Build history of the part. All positions in model axes, mm. A direction names the side the tool comes from. Give positions to 0.01 mm unless a question says otherwise; leave off trailing zeros. Loops run counter-clockwise (first coordinate to the right, second up) from the corner with the lowest first, then second, coordinate; pieces in that order, holes last. Notation, with made-up numbers: (5.5, 20.25) -> (32.5, 20.25) arc R25 ccw to (32.5, 47.25) -> close; hole circle Ø3 at (-2.5, 35). An arc over 180 degrees is marked (long way). Answer as a JSON object with one key per item and string values. Group by question number.
Q1. Band-saw the part on C-C, the plane z = 2. Write the cut outline in (x, y) (3 decimals), plus the area to 3 significant figures.
Q2. Wall check: probe 1 along Y at (x, z) = (0, 4.75) (3 decimals); probe 2 along Z at (x, y) = (1.5, -2.25); probe 3 along Y at (x, z) = (0, 1.5). Give the ranges that are in metal, low to high. Write a range as from..to.
Q3. Tool access for faces 1 (the cylindrical face through (0.25, -1.89, 3.94)), 2 (the cylindrical face through (-3.78, -2.9, 1.29)): list every direction of +Z, -Z, +X, -X, +Y, -Y with a clear straight run to the whole face (end or side of a thin tool).
from build123d import *

# Parameters (mm, degrees)
SKETCH1_R           = 4.7625
BOSS_EXTRUDE1_DEPTH = 1.5875
SKETCH3_R           = 1.905
BOSS_EXTRUDE2_DEPTH = 4.7625
SKETCH4_R           = 1.27
CUT_EXTRUDE1_DEPTH  = 10.256636133
CHAMFER2_SIZE       = 1


with BuildPart() as part:
    # Sketch1 → Boss-Extrude1 (new body)
    with BuildSketch(Plane.XY):
        Circle(SKETCH1_R)
    extrude(amount=BOSS_EXTRUDE1_DEPTH)

    # Sketch3 → Boss-Extrude2 (add)
    with BuildSketch(Plane.XY.offset(1.5875)):
        with Locations(Location((0, 0, 0), (0, 0, 180))):
            Circle(SKETCH3_R)
    extrude(amount=BOSS_EXTRUDE2_DEPTH)

    # Sketch4 → Cut-Extrude1 (cut, through all)
    with BuildSketch(Plane.XY.offset(6.35)):
        Circle(SKETCH4_R)
    extrude(amount=-CUT_EXTRUDE1_DEPTH, mode=Mode.SUBTRACT)

    # Chamfer2
    chamfer2_edges = [part.edges().sort_by_distance(p)[0] for p in [
        (-4.7625, 0, 0),
    ]]
    chamfer(chamfer2_edges, length=CHAMFER2_SIZE)


solid = part.part
Worked answers:
{
 "1": {"outline": "circle Ø3.81 at (0, 0); hole circle Ø2.54 at (0, 0)", "area": "6.33 mm2"},
 "2": {"probe 1": "-1.905..-1.27, 1.27..1.905", "probe 2": "0..1.59", "probe 3": "-4.76..-1.27, 1.27..4.76"},
 "3": {"face 1": "+Z", "face 2": "+Z, -Z"}
}
